Source: CAD feature listing. Evaluate the final solid. Frame: model axes, mm. Give positions to 0.01 mm unless a question says otherwise; leave off trailing zeros. Loops run counter-clockwise (first coordinate to the right, second up) from the corner with the lowest first, then second, coordinate; pieces in that order, holes last. Notation, with made-up numbers: (-19.75, 48) -> (31.25, 48) arc R33 cw to (31.25, 80) -> close; hole circle Ø5 at (77.5, -10.75). An arc over 180 degrees is marked (long way). Return JSON: item names as keys, results as strings. Group by question number.
(1) Cut plane C-C on x = 14.75. Return loops of the section in (y, z).
(2) Ray query, line 1 (Y direction, x = 6.25, z = 200); line 2 (Z direction, x = 10.25, y = 115.5). Return the intervals inside material, ascending. Write a range as from..to.
(3) Cut plane D-D on y = -105.5. Return loops of the section in (x, z).
(4) Pin query (flat end, axial travel): pin 1 (3 mm diameter, centred on y = -147.5, z = 65, fed in from +X). Return the tip coordinate at first contact, or that it passes through.
(5) Cut plane A-A on z = -200. Return loops of the section in (x, y).
(6) Draft query along Z for faces 1 (the face through (10, -250, 3)), 2 (the face through (10, -3, 3)), 3 (the face through (10, -3, -250)). Return one class per face: released by +Z, released by -Z, zero draft, split by the parting line, or undercut.
Autodesk Inventor part; units mm, degrees
ref_plane "YZ Plane" through (0, 0, 0) normal (1, 0, 0) x (0, 1, 0)
ref_plane "XZ Plane" through (0, 0, 0) normal (0, 1, 0) x (-1, 0, 0)
ref_plane "XY Plane" through (0, 0, 0) normal (0, 0, 1) x (1, 0, 0)
sketch "Sketch1" plane through (0, 0, 0) normal (1, 0, 0) x (0, 1, 0)
  line L0 (250, 250) -> (-250, 250)
  line L1 (-250, 250) -> (-250, -250)
  line L2 (-250, -250) -> (250, -250)
  line L3 (250, -250) -> (250, 250)
  line L4 (250, 250) -> (-250, -250) construction
  line L5 (-250, 250) -> (250, -250) construction
  point P0 (0, 0)
  dimension "d0" = 500
  dimension "d1" = 500
extrude "Extrusion1" add sketch "Sketch1" along normal blind 10
sketch "Sketch2" plane through (10, 0, 0) normal (1, 0, 0) x (0, 0, -1)
  line L0 (-250, 250) -> (-250, -250)
  line L1 (-250, -250) -> (250, -250)
  line L2 (250, -250) -> (250, 250)
  line L3 (250, 250) -> (-250, 250)
  line L4 (-230, 230) -> (230, 230)
  line L5 (230, 230) -> (230, -230)
  line L6 (230, -230) -> (-230, -230)
  line L7 (-230, -230) -> (-230, 230)
  line L8 (-230, 230) -> (230, -230) construction
  line L9 (230, 230) -> (-230, -230) construction
  point P0 (0, 0)
  dimension "d4" = 20
  dimension "d5" = 20
extrude "Extrusion2" add sketch "Sketch2" along normal blind 10
sketch "Sketch3" plane through (10, 0, 0) normal (1, 0, 0) x (0, 0, -1)
  circle A0 centre (-200, -200) radius 30
  line L0 (-250, 250) -> (-250, -250)
  line L1 (-250, -250) -> (250, -250)
  point P0 (0, 0)
  dimension "d8" = 60
  dimension "d9" = 50
  dimension "d10" = 50
hole "Hole1" at (10, -200, 200) direction (-1, 0, 0) diameter 30 depth 67.75
mirror "Mirror1" about plane through (0, 0, 0) normal (0, 1, 0) of "Hole1"
mirror "Mirror2" about plane through (0, 0, 0) normal (0, 0, 1) of "Hole1", "Mirror1"
sketch "Sketch4" plane through (10, 0, 0) normal (1, 0, 0) x (0, 0, -1)
  line L0 (-250, 250) -> (254.1843, 248.5364) construction
  line L1 (254.1843, 248.5364) -> (252.7352, -250.6505) construction
  line L2 (252.7352, -250.6505) -> (-251.4491, -249.1869) construction
  line L3 (-251.4491, -249.1869) -> (-250, 250) construction
  point P0 (0, 0)
properties part number "S.Carrom board" material "Birch"
Answers:
{
 "1": {"outline": "(-250, -250) -> (250, -250) -> (250, 250) -> (-250, 250) -> close; hole (-230, -230) -> (230, -230) -> (230, 230) -> (-230, 230) -> close"},
 "2": {"line 1": "-250..-215, -185..185, 215..250", "line 2": "-250..-230, 230..250"},
 "3": {"outline": "(0, -250) -> (20, -250) -> (20, -230) -> (10, -230) -> (10, 230) -> (20, 230) -> (20, 250) -> (0, 250) -> close"},
 "4": {"pin 1": "x = 10"},
 "5": {"outline": "(0, -250) -> (20, -250) -> (20, -230) -> (10, -230) -> (10, -215) -> (0, -215) -> close; (0, -185) -> (10, -185) -> (10, 185) -> (0, 185) -> close; (0, 215) -> (10, 215) -> (10, 230) -> (20, 230) -> (20, 250) -> (0, 250) -> close"},
 "6": {"face 1": "zero draft", "face 2": "undercut", "face 3": "released by -Z"}
}
